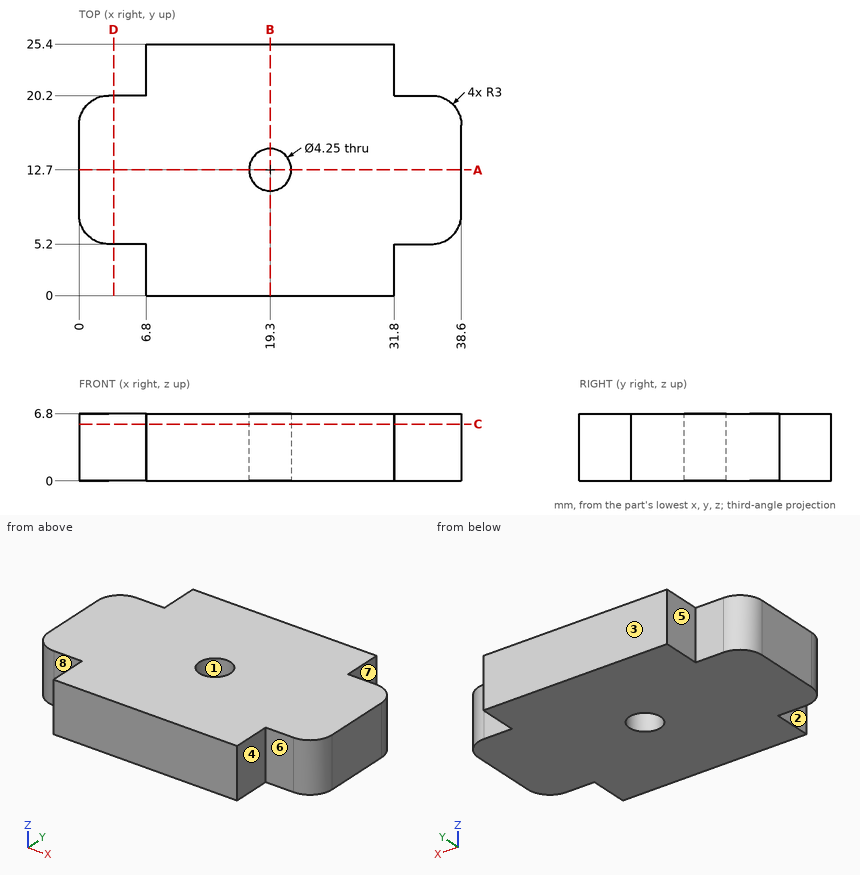
Print and shaded views of the part. All mm, measured from the part's lowest x, y and z. A direction names the side the tool comes from. Round coordinates to 2 decimals unless told otherwise and drop trailing zeros. Write each loop counter-clockwise with the first axis right and the second up, starting at its lowest first coordinate (ties: lowest second). Pieces come first, ordered by that corner, then holes. Notation, with made-up numbers: (-32.75, 76.25) -> (16.25, 76.25) arc R5 ccw to (16.25, 85.25) -> close; hole circle Ø2 at (-28.5, 34.25). An arc over 180 degrees is marked (long way). Write item = value, one per line.
(1) Tool access for the marked faces 5, 6, 7 and 8: list every direction of +Z, -Z, +X, -X, +Y, -Y with a clear straight run to the whole face (end or side of a thin tool).
Answer:
face_5 = +Z, -Z, -X, +Y
face_6 = +Z, -Z, +X, -Y
face_7 = +Z, -Z, +X, +Y
face_8 = +Z, -Z, -X, -Y
(2) Flat gauge pins, fed straight in: pin 1 (1.1 mm diameter, centred on x = 5.5, z = 4.5, fed in from -Y); pin 2 (4 mm diameter, centred on y = 1.5, z = 4.5, fed in from +X); pin 3 (4 mm diameter, centred on y = 2.5, z = 4.5, fed in from -X). Where does each tip first touch, or does it go through?
Answer:
pin_1 = 5.2
pin_2 = 31.8
pin_3 = 6.8
(3) Band-saw the part on C-C (z = 5.75). Give the cut face in (x, y) (3 decimals).
Answer:
outline = (0, 8.2) arc R3 ccw to (3, 5.2) -> (6.8, 5.2) -> (6.8, 0) -> (31.8, 0) -> (31.8, 5.2) -> (35.6, 5.2) arc R3 ccw to (38.6, 8.2) -> (38.6, 17.2) arc R3 ccw to (35.6, 20.2) -> (31.8, 20.2) -> (31.8, 25.4) -> (6.8, 25.4) -> (6.8, 20.2) -> (3, 20.2) arc R3 ccw to (0, 17.2) -> close; hole circle Ø4.25 at (19.3, 12.7)
(4) Band-saw the part on B-B (x = 19.3). Give the cut face in (y, z) (3 decimals).
Answer:
outline = (0, 0) -> (10.575, 0) -> (10.575, 6.8) -> (0, 6.8) -> close; (14.825, 0) -> (25.4, 0) -> (25.4, 6.8) -> (14.825, 6.8) -> close
(5) Probe L1, parallel to Y at x = 19.3, z = 2.25 (3 decimals); L2, parallel to X at y = 22.75, z = 5.5; L3, parallel to X at y = 7.75, z = 4. List the from-to ranges inside material, lowest first.
Answer:
L1 = 0 to 10.575, 14.825 to 25.4
L2 = 6.8 to 31.8
L3 = 0.03 to 38.57
(6) Band-saw the part on D-D (x = 3.5). Give the cut face in (y, z).
Answer:
outline = (5.2, 0) -> (20.2, 0) -> (20.2, 6.8) -> (5.2, 6.8) -> close
(7) Two-plate mould, pull along X, no slides. Class the marked faces 1, 2, 3 and 4: pulls with the +X half, pulls with the -X half, needs draft (parallel to the pull), parting line crosses it, or undercut.
Answer:
face_1 = undercut
face_2 = pulls with the -X half
face_3 = needs draft
face_4 = pulls with the +X half
(8) Band-saw the part on A-A (y = 12.7). Give the cut face in (x, z) (3 decimals), then the cut area to 3 significant figures.
Answer:
outline = (0, 0) -> (17.175, 0) -> (17.175, 6.8) -> (0, 6.8) -> close; (21.425, 0) -> (38.6, 0) -> (38.6, 6.8) -> (21.425, 6.8) -> close
area = 234 mm2
